Verification items for the finished model (mm, model axes). A direction names the side the tool comes from. Coordinates: 2 decimals unless noted, no trailing zeros. Order: outer loops, then holes, each group sorted by start corner. A loop starts at its lowest first (then second) coordinate and runs counter-clockwise, first axis right, second up. Notation, with made-up numbers: (13, 45) -> (60, 45) arc R28 ccw to (60, 73) -> close; hole circle Ø6 at (29.25, -34.75). An arc over 180 degrees is marked (long way). Use CSV: the item, a comma, the result in double quotes. Start each with the question number.
1) Scan lines: line 1 along X through (y, z) = (-300, 743); line 2 along X through (y, z) = (-291, 715.5); line 3 along Y through (x, z) = (1480, 734.25). Record each from-to range of solid material in increasing order.
2) Tool access check on faces 1 (the flat face through (740, -280, 734)), 2 (the flat face through (25, -305, 730)), 3 (the flat face through (755, -305, 730)), 4 (the flat face through (1485, -305, 730)). Record the directions out of +Z, -Z, +X, -X, +Y, -Y that give a thin tool (end or side, any length) a straight path to the whole face; none if there is none.
3) Sectioned sample at A-A on z = 722. Record the boundary of the cut face in (x, y), then the cut area to 3 significant figures.
4) Go/stop test with flat-tipped pins: pin 1 (10 mm diameter, centred on y = -302.5, z = 724, fed in from +X); pin 2 (20 mm diameter, centred on x = 23.5, y = -305.5, fed in from -Z); pin 3 (22 mm diameter, centred on y = -296.5, z = 717.5, fed in from -X); pin 4 (6 mm diameter, centred on x = 20, y = -300, fed in from +Z). Record where each tip stops, or that it passes through.
from build123d import *

# Parameters (mm, degrees)
SKETCH030_W     = 40
SKETCH030_H     = 40
PAD022_DEPTH    = 1500
SKETCH031_W     = 40
SKETCH031_H     = 40
POCKET008_DEPTH = 20
SKETCH059_R     = 5
POCKET014_DEPTH = 40.001


with BuildPart() as part:
    # Sketch030 → Pad022 (new body)
    with BuildSketch(Plane.YZ):
        with Locations((-300, 280)):
            Rectangle(SKETCH030_W, SKETCH030_H)
    extrude(amount=PAD022_DEPTH)

    # Sketch031 (on Face3 of Pad022) → Pocket008 (cut)
    with BuildSketch(Plane.YX.offset(-260)):
        with Locations((-300, 1480)):
            Rectangle(SKETCH031_W, SKETCH031_H)
        with Locations((-300, 750)):
            Rectangle(SKETCH031_W, SKETCH031_H)
        with Locations((-300, 20)):
            Rectangle(SKETCH031_W, SKETCH031_H)
    extrude(amount=-POCKET008_DEPTH, mode=Mode.SUBTRACT)

    # Sketch059 → Pocket014 (cut, through all)
    with BuildSketch(Plane(origin=(0, 0, 300), x_dir=(0, -1, 0), z_dir=(0, 0, 1))):
        with Locations((300, 20)):
            Circle(SKETCH059_R)
        with Locations((300, 750)):
            Circle(SKETCH059_R)
        with Locations((300, 1480)):
            Circle(SKETCH059_R)
    extrude(amount=-POCKET014_DEPTH, mode=Mode.SUBTRACT)


with BuildPart() as part_1:
    # Clone010 placement: moved
    add(part.part.moved(Location((0, 0, 450))))


solid = part_1.part
Answers follow:
1,line 1,"x = 0 to 15, 25 to 745, 755 to 1475, 1485 to 1500"
1,line 2,"x = 40 to 730, 770 to 1460"
1,line 3,"y = -320 to -305, -295 to -280"
2,face 1,"+Z, -Z, +X, -X, +Y"
2,face 2,"-Z, -X, +Y, -Y"
2,face 3,"-Z, +Y, -Y"
2,face 4,"-Z, +X, +Y, -Y"
3,outline,"(40, -320) -> (730, -320) -> (730, -280) -> (40, -280) -> close; (770, -320) -> (1460, -320) -> (1460, -280) -> (770, -280) -> close"
3,area,"55,200 mm²"
4,pin 1,"stops at x = 1460"
4,pin 2,"stops at z = 730"
4,pin 3,"stops at x = 40"
4,pin 4,"passes through"
